The listing builds one solid part. Answer for the finished solid, in the listing's coordinates (mm). A direction names the side the tool comes from. Coordinates: 2 decimals unless noted, no trailing zeros. Order: outer loops, then holes, each group sorted by start corner. A loop starts at its lowest first (then second) coordinate and runs counter-clockwise, first axis right, second up. Notation, with made-up numbers: (-31, 51) - (3, 51) arc R38 cw to (3, 89) - close; hole circle Ø4 at (-5.75, 72.25). An arc over 180 degrees is marked (long way). One line per item, written item: value. Start each with the question number.
```python
from build123d import *

# Parameters (mm, degrees)
RESSALTO_EXTRUS_O1_DEPTH = 10
ESBO_O2_R                = 1.5
CORTE_EXTRUS_O1_DEPTH    = 11
RESSALTO_EXTRUS_O2_DEPTH = 10
ESBO_O4_W                = 4
ESBO_O4_H                = 5
CORTE_EXTRUS_O4_DEPTH    = 44
ESBO_O5_W                = 10
ESBO_O5_H                = 5
RESSALTO_EXTRUS_O3_DEPTH = 10
ESBO_O6_W                = 10
ESBO_O6_H                = 10
RESSALTO_EXTRUS_O4_DEPTH = 5
FURO_COM_FOLGA_DE_M41_D  = 4.5


with BuildPart() as part:
    # Esboço1 → Ressalto-extrusão1 (new body)
    with BuildSketch(Plane(origin=(0, 0, 0), x_dir=(1, 0, 0), z_dir=(0, 1, 0))):
        Polygon((-21.5, 0), (-21.5, -23), (-11.5, -23), (-11.5, -10), (11.5, -10), (11.5, -23), (21.5, -23), (21.5, 0), align=None)
    extrude(amount=RESSALTO_EXTRUS_O1_DEPTH)

    # Esboço2 → Corte-extrusão1 (cut, through all)
    with BuildSketch(Plane(origin=(0, 10, 0), x_dir=(1, 0, 0), z_dir=(0, 1, 0))):
        with Locations((-13.9, -16.5)):
            Circle(ESBO_O2_R)
        with Locations((13.9, -16.5)):
            Circle(ESBO_O2_R)
    extrude(amount=-CORTE_EXTRUS_O1_DEPTH, mode=Mode.SUBTRACT)

    # Esboço3 → Ressalto-extrusão2 (add)
    with BuildSketch(Plane(origin=(0, 10, 0), x_dir=(1, 0, 0), z_dir=(0, 1, 0))):
        Polygon((-21.5, -23), (-21.5, -27), (-21.5, -32), (-11.5, -32), (-11.5, -27), (-11.5, -23), align=None)
        Polygon((11.5, -23), (21.5, -23), (21.5, -27), (21.5, -32), (11.5, -32), (11.5, -27), align=None)
    extrude(amount=-RESSALTO_EXTRUS_O2_DEPTH)

    # Esboço4 → Corte-extrusão4 (cut, through all)
    with BuildSketch(Plane(origin=(21.5, 0, 0), x_dir=(0, 0, -1), z_dir=(1, 0, 0))):
        with Locations((-25, 2.5)):
            Rectangle(ESBO_O4_W, ESBO_O4_H)
    extrude(amount=-CORTE_EXTRUS_O4_DEPTH, mode=Mode.SUBTRACT)

    # Esboço5 → Ressalto-extrusão3 (add)
    with BuildSketch(Plane.XZ):
        with Locations((-16.5, 29.5)):
            Rectangle(ESBO_O5_W, ESBO_O5_H)
        with Locations((16.5, 29.5)):
            Rectangle(ESBO_O5_W, ESBO_O5_H)
    extrude(amount=RESSALTO_EXTRUS_O3_DEPTH)

    # Esboço6 → Ressalto-extrusão4 (add)
    with BuildSketch(Plane.XY.offset(32)):
        with Locations((-26.5, -5)):
            Rectangle(ESBO_O6_W, ESBO_O6_H)
        with Locations((26.5, -5)):
            Rectangle(ESBO_O6_W, ESBO_O6_H)
    extrude(amount=-RESSALTO_EXTRUS_O4_DEPTH)

    # Furo com folga de M41 (through all)
    with Locations(Plane(origin=(-26.5, -5, 32), x_dir=(1, 0, 0), z_dir=(0, 0, 1))):
        with Locations((0, 0), (53, 0)):
            Hole(FURO_COM_FOLGA_DE_M41_D / 2)


solid = part.part
```
(1) For a pull along X with two mould halves and no side action, classify faces 4 (the face through (21, -10, 30)), 5 (the face through (-21.5, 5, 16)), 6 (the face through (-15.4, 5.07, 16.43)) as pulls with the +X half, pulls with the -X half, needs draft (parallel to the pull), parting line crosses it, or undercut.
(2) The part is cut by section B-B on x = -13.9. Determine the outline of the cut face in (y, z), plus the area to 3 significant figures.
(3) Consider probe 1 along X at (y, z) = (5, 16.5); probe 2 along X at (y, z) = (4.5, 14); probe 3 along Z at (x, y) = (17.5, 3.25). Determine where each line is inside the solid, lowest interval first.
(4) The part is cut by section D-D on y = 8. Determine the outline of the cut face in (x, z), plus the area to 3 significant figures.
(5) Flat-ended cylindrical pins translate along their axes: pin 1 Ø4 at (x, z) = (-26, 29) entering from +Y; pin 2 Ø1.5 at (y, z) = (-1.5, 5.5) entering from +X; pin 3 Ø5 at (x, y) = (26.5, -5) entering from +Z; pin 4 Ø3 at (y, z) = (5.5, 9.5) entering from -X. Find the tip coordinate at first contact, or state that the pin passes through.
(6) The part is cut by section A-A on y = 3.75. Determine the outline of the cut face in (x, z), plus the area to 3 significant figures.
(7) For faces 1 (the face through (0, 0, 9)), 2 (the face through (17, 2, 23)), 3 (the face through (0, 5, 10)), determine the directions among +Z, -Z, +X, -X, +Y, -Y from which every point of the face is accessible in a straight line to the end or side of a thin tool.
(8) The part is cut by section C-C on z = 20. Determine the outline of the cut face in (x, y).
Completed:
1. face 4: needs draft
1. face 5: pulls with the -X half
1. face 6: undercut
2. outline: (-10, 27) - (5, 27) - (5, 23) - (0, 23) - (0, 18) - (10, 18) - (10, 32) - (-10, 32) - close; (0, 0) - (10, 0) - (10, 15) - (0, 15) - close
2. area: 320 mm2
3. probe 1: x = -21.5 to -15.4, -12.4 to -11.5, 11.5 to 12.4, 15.4 to 21.5
3. probe 2: x = -21.5 to -11.5, 11.5 to 21.5
3. probe 3: z = 0 to 23, 27 to 32
4. outline: (-21.5, 0) - (21.5, 0) - (21.5, 32) - (11.5, 32) - (11.5, 10) - (-11.5, 10) - (-11.5, 32) - (-21.5, 32) - close; hole circle Ø3 at (-13.9, 16.5); hole circle Ø3 at (13.9, 16.5)
4. area: 856 mm2
5. pin 1: stops at y = 0
5. pin 2: passes through
5. pin 3: stops at z = 32
5. pin 4: stops at x = -21.5
6. outline: (-21.5, 0) - (21.5, 0) - (21.5, 23) - (11.5, 23) - (11.5, 10) - (-11.5, 10) - (-11.5, 23) - (-21.5, 23) - close; (-21.5, 27) - (-11.5, 27) - (-11.5, 32) - (-21.5, 32) - close; (11.5, 27) - (21.5, 27) - (21.5, 32) - (11.5, 32) - close; hole circle Ø3 at (-13.9, 16.5); hole circle Ø3 at (13.9, 16.5)
6. area: 776 mm2
7. face 1: -Z, +X, -X, -Y
7. face 2: +X, -X, -Y
7. face 3: +Z, +Y, -Y
8. outline: (-21.5, 0) - (-11.5, 0) - (-11.5, 10) - (-21.5, 10) - close; (11.5, 0) - (21.5, 0) - (21.5, 10) - (11.5, 10) - close
